Source: CAD feature listing. Evaluate the final solid. Frame: model axes, mm. Face numbers are marked on the shaded views. A direction names the side the tool comes from. Coordinates: 2 decimals unless noted, no trailing zeros. Loops run counter-clockwise (first coordinate to the right, second up) from the corner with the lowest first, then second, coordinate; pieces in that order, holes last.
Item 1: Section query D-D, the plane y = 5.5. Return the cut outline in (x, z), then the cut area to 3 significant figures.
Item 2: Section query A-A, the plane z = 0. Return the cut outline in (x, y), then the cut area to 3 significant figures.
Item 3: Line query: probe 1 along Z at (x, y) = (9.5, 8.25); probe 2 along X at (y, z) = (7.75, 13); probe 3 along X at (y, z) = (9.25, -44). Output: solid intervals per line, ascending.
Item 4: Reachability of the marked faces 1 and 2 from +Z, -Z, +X, -X, +Y, -Y: full face, straight path, thin tool, end or side. Return the list, or none.
Item 5: Section query C-C, the plane z = -19. Return the cut outline in (x, y).
Item 6: Pin query (flat end, axial travel): pin 1 Ø3 at (y, z) = (4.5, -28) entering from -X; pin 2 Ø2 at (y, z) = (5.5, 5) entering from -X; pin 3 Ø3 at (y, z) = (2.5, -9.5) entering from -X; pin 4 Ø3 at (x, z) = (-43.5, -48) entering from -Y. Return the tip coordinate at first contact, or that it passes through.
Item 7: Pull-direction query (X, two-part tool) for the marked faces 3, 4 and 5; classes: +X half, -X half, draft (parallel to the pull), parting line (faces both ways), or undercut.
Item 8: Section query B-B, the plane x = -46. Return the cut outline in (y, z), then the cut area to 3 significant figures.
Autodesk Inventor part; units mm, degrees
ref_plane "YZ Plane" through (0, 0, 0) normal (1, 0, 0) x (0, 1, 0)
ref_plane "XZ Plane" through (0, 0, 0) normal (0, 1, 0) x (-1, 0, 0)
ref_plane "XY Plane" through (0, 0, 0) normal (0, 0, 1) x (1, 0, 0)
sketch "Sketch1" plane through (0, 0, 0) normal (0, 1, 0) x (-1, 0, 0)
  circle A0 centre (0, 0) radius 62.2958
  line L0 (-0.7, -10) -> (0.7, -10)
  line L1 (0.6998, 10) -> (-0.7, 10)
  line L2 (0.7, -10) -> (0.7, -2.8135)
  line L3 (0.6998, 2.8135) -> (0.6998, 10)
  line L4 (-0.7, 10) -> (-0.7, 2.8142)
  line L5 (-0.7, -2.8142) -> (-0.7, -10)
  arc A1 (-0.7, 2.8142) -> (-0.7, -2.8142) centre (0, 0) ccw
  arc A2 (0.7, -2.8135) -> (0.6998, 2.8135) centre (0, 0) ccw
  dimension "d0" = 124.5916
  dimension "d2" = 1.4
  dimension "d6" = 20
  dimension "d7" = 10
extrude "Extrusion1" add sketch "Sketch1" along normal blind 10
sketch "Sketch4" plane through (0, 0, 0) normal (0, -1, 0) x (1, 0, 0)
  point P0 (0, 0)
sketch "Sketch6" plane through (0, 0, 0) normal (0, -1, 0) x (1, 0, 0)
  circle A0 centre (0, 0) radius 17.5
  line L0 (70.933, -2.5) -> (70.933, 2.5)
  line L1 (-76.7315, 1.75) -> (-76.7315, -1.75)
  arc A1 (-0.6998, 2.8135) -> (-0.7, -2.8135) centre (0, 0) ccw
  arc A2 (0.7, -2.8142) -> (0.7, 2.8142) centre (0, 0) ccw
  circle A3 centre (0, 0) radius 55
  line L2 (2.5, 115.1017) -> (-2.5, 115.1017)
  line L3 (-2.5, -115.1017) -> (2.5, -115.1017)
  line L4 (0.7, 10) -> (-0.6998, 10)
  circle A4 centre (0, 0) radius 62.2958
  line L5 (-76.7315, -1.75) -> (-17.4123, -1.75)
  line L6 (-17.4123, 1.75) -> (-76.7315, 1.75)
  line L7 (-1.4682, 2.5) -> (-1.4697, 2.5)
  line L8 (-1.75, -17.4123) -> (-1.75, -76.7315)
  line L9 (1.75, -76.7315) -> (1.75, -17.4123)
  line L10 (17.4123, -1.75) -> (76.7315, -1.75)
  line L11 (76.7315, 1.75) -> (17.4123, 1.75)
  line L12 (1.75, 17.4123) -> (1.75, 76.7315)
  line L13 (-1.75, 76.7315) -> (-1.75, 17.4123)
  point P0 (-2.8993, 0)
  point P1 (-2.5, 17.3205)
  point P2 (-2.5, -17.3205)
  point P3 (2.5, -17.3205)
  point P4 (17.3205, -2.5)
  point P5 (17.3205, 2.5)
  point P6 (2.5, 17.3205)
  point P7 (-54.9722, 1.75)
  point P8 (-54.9722, -1.75)
  point P9 (54.9722, -1.75)
  point P10 (1.75, -54.9722)
  point P11 (1.75, 54.9722)
  point P12 (54.9722, 1.75)
  point P13 (-1.75, 54.9722)
  point P14 (-1.75, -54.9722)
  dimension "d16" = 35
  dimension "d18" = 110
  dimension "d19" = 5
  dimension "d22" = 1.75
  dimension "d23" = 3.5
  dimension "d26" = 360
extrude "Extrusion2" cut sketch "Sketch6" against normal blind 10 contours A0 L12 A3 L11 | L10 A3 L9 A0 | A0 L6 A3 L13 | L8 A3 L5 A0
properties part number "Pot Disk"
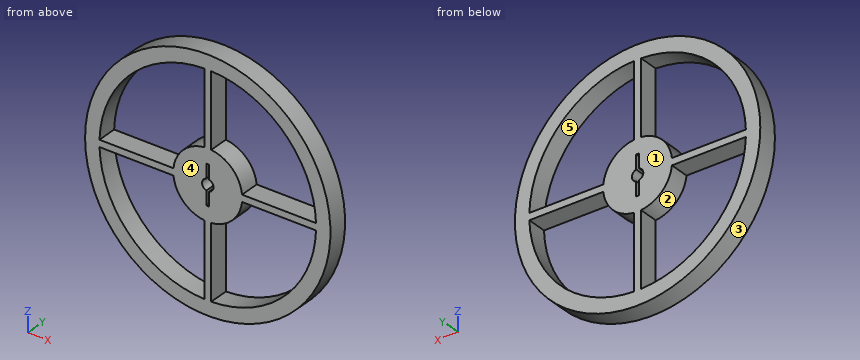
Verdict:
1. outline: circle Ø124.59 at (0, 0); hole (-54.97, -1.75) arc R55 ccw to (-1.75, -54.97) - (-1.75, -17.41) arc R17.5 cw to (-17.41, -1.75) - close; hole (-54.97, 1.75) - (-17.41, 1.75) arc R17.5 cw to (-1.75, 17.41) - (-1.75, 54.97) arc R55 ccw to start; hole (-0.7, -10) - (0.7, -10) - (0.7, -2.81) arc R2.9 ccw to (0.7, 2.81) - (0.7, 10) - (-0.7, 10) - (-0.7, 2.81) arc R2.9 ccw to (-0.7, -2.81) - close; hole (1.75, -54.97) arc R55 ccw to (54.97, -1.75) - (17.41, -1.75) arc R17.5 cw to (1.75, -17.41) - close; hole (1.75, 17.41) arc R17.5 cw to (17.41, 1.75) - (54.97, 1.75) arc R55 ccw to (1.75, 54.97) - close
1. area: 4,130 mm2
2. outline: (-62.3, 0) - (-2.9, 0) - (-2.9, 10) - (-62.3, 10) - close; (2.9, 0) - (62.3, 0) - (62.3, 10) - (2.9, 10) - close
2. area: 1,190 mm2
3. probe 1: z = -61.57 to -54.17, -14.7 to 14.7, 54.17 to 61.57
3. probe 2: x = -60.92 to -53.44, -11.72 to 11.72, 53.44 to 60.92
3. probe 3: x = -44.1 to -33, -1.75 to 1.75, 33 to 44.1
4. face 1: +Z, -Z, +X, -X, +Y
4. face 2: +Y, -Y
5. outline: (-59.33, 0) - (-51.61, 0) - (-51.61, 10) - (-59.33, 10) - close; (-1.75, 0) - (1.75, 0) - (1.75, 10) - (-1.75, 10) - close; (51.61, 0) - (59.33, 0) - (59.33, 10) - (51.61, 10) - close
6. pin 1: stops at x = -56.38
6. pin 2: stops at x = -62.17
6. pin 3: stops at x = -61.78
6. pin 4: passes through
7. face 3: parting line
7. face 4: draft
7. face 5: undercut
8. outline: (0, -42.01) - (10, -42.01) - (10, -30.15) - (0, -30.15) - close; (0, -1.75) - (10, -1.75) - (10, 1.75) - (0, 1.75) - close; (0, 30.15) - (10, 30.15) - (10, 42.01) - (0, 42.01) - close
8. area: 272 mm2
